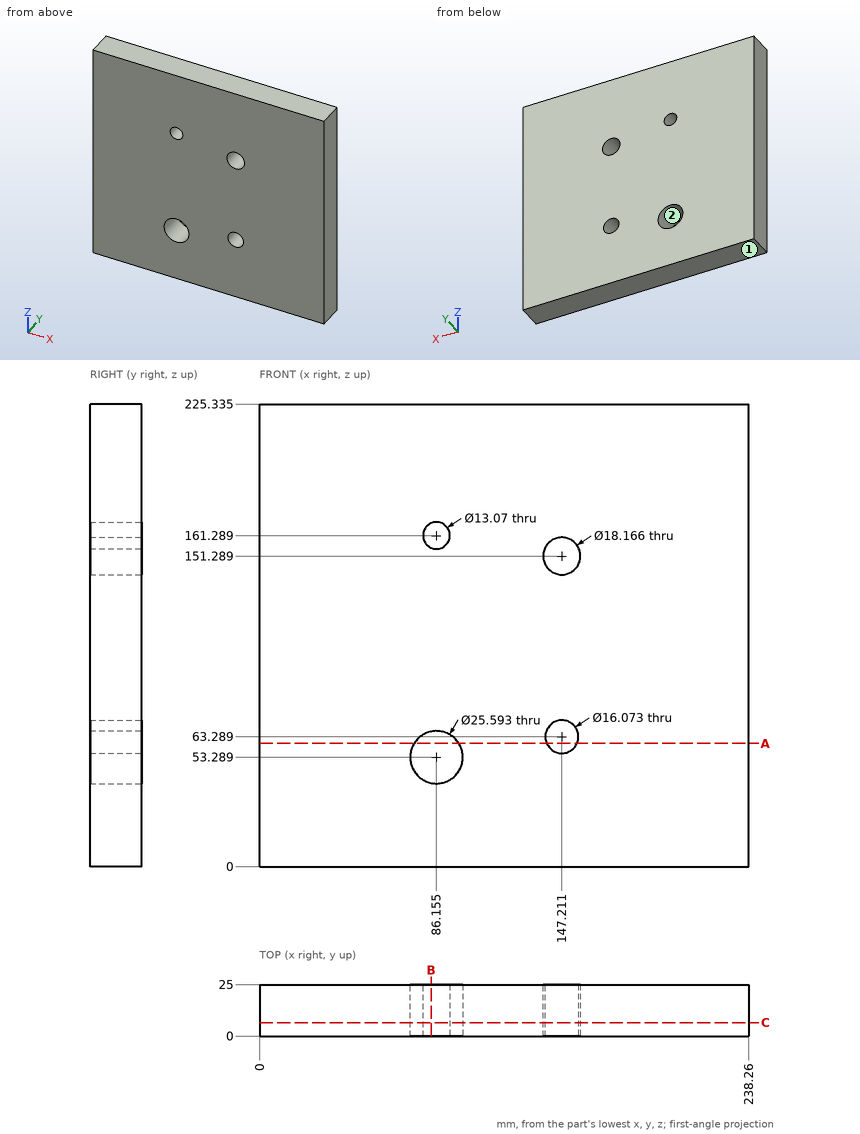
Print and shaded views of the part. All mm, measured from the part's lowest x, y and z. Give positions to 0.01 mm unless a question says otherwise; leave off trailing zeros. Loops run counter-clockwise (first coordinate to the right, second up) from the corner with the lowest first, then second, coordinate; pieces in that order, holes last. Notation, with made-up numbers: M 32,2 L 73,2 A14 ccw 73,16 Z; hole C 51.25,7 d2. An arc over 180 degrees is marked long. Write each question's results on one line, items separated by ' | '.
Q1. Band-saw the part on A-A on z = 60. Write the cut outline in (x, y).
Geometry check:
outline: M 0,0 L 75.26,0 L 75.26,25 L 0,25 Z; M 97.05,0 L 139.88,0 L 139.88,25 L 97.05,25 Z; M 154.54,0 L 238.26,0 L 238.26,25 L 154.54,25 Z
Q2. Band-saw the part on C-C on y = 6.5. Write the cut outline in (x, z) (1 decimal).
Geometry check:
outline: M 0,0 L 238.3,0 L 238.3,225.3 L 0,225.3 Z; hole C 86.2,53.3 d25.6; hole C 86.2,161.3 d13.1; hole C 147.2,151.3 d18.2; hole C 147.2,63.3 d16.1
Q3. Flat gauge pin, fed straight in: P1, Ø8, axis at x = 86.15, z = 161.29, coming from the +Y side. Where does the tip first touch, or does it go through?
Geometry check:
P1: passes through
Q4. Mould opens along X. For the marked faces 1 and 2 say: pulls with the +X half, pulls with the -X half, needs draft (parallel to the pull), parting line crosses it, or undercut.
Geometry check:
face 1: needs draft | face 2: undercut
Q5. Probe probe 1 along Z at (x, y) = (147.5, 17.5) (1 decimal); probe 2 along Z at (x, y) = (82, 6.75) (1 decimal); probe 3 along X at (y, z) = (10, 47). List the from-to ranges inside material, lowest first.
Geometry check:
probe 1: z = 0 to 55.3, 71.3 to 142.2, 160.4 to 225.3 | probe 2: z = 0 to 41.2, 65.4 to 156.2, 166.3 to 225.3 | probe 3: x = 0 to 75.01, 97.3 to 238.26
Q6. Band-saw the part on B-B on x = 83.5. Write the cut outline in (y, z) (1 decimal).
Geometry check:
outline: M 0,0 L 25,0 L 25,40.8 L 0,40.8 Z; M 0,65.8 L 25,65.8 L 25,155.3 L 0,155.3 Z; M 0,167.3 L 25,167.3 L 25,225.3 L 0,225.3 Z
